Read the model definition and answer for the solid it produces. Units are mm, in the model's axes. A direction names the side the tool comes from. Coordinates: 2 decimals unless noted, no trailing zeros. Loops run counter-clockwise (first coordinate to the right, second up) from the corner with the lowest first, then second, coordinate; pieces in that order, holes last. Notation, with made-up numbers: M 77,-28 L 115,-28 A28 cw 115,-6 Z; hole C 33,-39 d8. An arc over 180 degrees is marked long. One line per item, written item: value. Start each with the question number.
```python
from build123d import *

# Parameters (mm, degrees)
F0_W      = 60
F0_H      = 88
F1_DEPTH  = 34
F3_DEPTH  = 58
F4_W      = 13
F4_H      = 5
F5_DEPTH  = 33
F7_DEPTH  = 1.001
F9_DEPTH  = 2.001
F4_W_2    = 58
F4_H_2    = 10
F10_DEPTH = 25
F11_W     = 58
F11_H     = 7
F12_DEPTH = 10
F14_DEPTH = 3
F15_R     = 1.75
F16_DEPTH = 3


with BuildPart() as f1:
    # F0 (on Front) → F1 (new body)
    with BuildSketch(Plane.XZ):
        Rectangle(F0_W, F0_H)
    extrude(amount=F1_DEPTH)

    # F2 (on face) → F3 (cut)
    with BuildSketch(Plane(origin=(-30, 0, 0), x_dir=(0, -1, 0), z_dir=(-1, 0, 0))):
        Polygon((34, 39), (34, 44), (10, 44), (17, 39), align=None)
    extrude(amount=-F3_DEPTH, mode=Mode.SUBTRACT)

    # F4 (on face) → F5 (cut)
    with BuildSketch(Plane.XZ.offset(34)):
        with Locations((-23.5, 41.5)):
            Rectangle(F4_W, F4_H)
    extrude(amount=-F5_DEPTH, mode=Mode.SUBTRACT)

    # F6 (on face) → F7 (cut, through all)
    with BuildSketch(Plane.XZ.offset(1)):
        with BuildLine():
            Line((-23.831531967, 44), (-23.7494568899, 40.7064042404))
            ThreePointArc((-23.7494568899, 40.7064042404), (-23.2219262295, 39.4972445212), (-22, 39))
            ThreePointArc((-22, 39), (-20.7625631329, 39.5125631329), (-20.25, 40.75))
            Line((-20.25, 40.75), (-20.25, 44))
            Line((-20.25, 44), (-23.831531967, 44))
        make_face()
    extrude(amount=-F7_DEPTH, mode=Mode.SUBTRACT)

    # F8 (on face) → F9 (cut, through all)
    with BuildSketch(Plane(origin=(28, 0, 0), x_dir=(0, -1, 0), z_dir=(-1, 0, 0))):
        with BuildLine():
            Line((24.25, 44), (24.25, 40.75))
            ThreePointArc((24.25, 40.75), (24.7625631329, 39.5125631329), (26, 39))
            ThreePointArc((26, 39), (27.2374368671, 39.5125631329), (27.75, 40.75))
            Line((27.75, 40.75), (27.75, 44))
            Line((27.75, 44), (24.25, 44))
        make_face()
    extrude(amount=-F9_DEPTH, mode=Mode.SUBTRACT)

    # F4 (on face) → F10 (cut)
    with BuildSketch(Plane.XZ.offset(34)):
        with Locations((-1, -39)):
            Rectangle(F4_W_2, F4_H_2)
    extrude(amount=-F10_DEPTH, mode=Mode.SUBTRACT)

    # F11 (on face) → F12 (cut)
    with BuildSketch(Plane(origin=(0, 0, -44), x_dir=(1, 0, 0), z_dir=(0, 0, -1))):
        with Locations((-1, 4.5)):
            Rectangle(F11_W, F11_H)
    extrude(amount=-F12_DEPTH, mode=Mode.SUBTRACT)

    # F13 (on face) → F14 (cut)
    with BuildSketch(Plane.XZ.offset(9)):
        with BuildLine():
            Line((21, -37), (21, -44))
            Line((21, -44), (28, -44))
            Line((28, -44), (28, -35))
            Line((28, -35), (23, -35))
            ThreePointArc((23, -35), (21.5857864376, -35.5857864376), (21, -37))
        make_face()
    extrude(amount=-F14_DEPTH, mode=Mode.SUBTRACT)

    # F15 (on face) → F16 (cut)
    with BuildSketch(Plane(origin=(0, 0, 0), x_dir=(-1, 0, 0), z_dir=(0, 1, 0))):
        with Locations((-25.15, -40.15)):
            Circle(F15_R)
    extrude(amount=-F16_DEPTH, mode=Mode.SUBTRACT)


solid = f1.part
```
1) Section B-B (z = -40.15) is taken. Determine the outline of the cut face in (x, y), then the cut area to 4 significant figures.
2) Section C-C (x = 8.5) is taken. Determine the outline of the cut face in (y, z).
3) For a pull along X with two mould halves and no side action, classify faces 1 (the face through (5, -7, 44)), 2 (the face through (-30, -17, -1)), 3 (the face through (24.34, -0.49, -41.7)), 4 (the face through (21.6, -8.51, -35.57)) as released by +X, released by -X, zero draft, split by the parting line, or undercut.
4) Consider line 1 along Z through (x, y) = (25.15, -0.25); line 2 along Y through (x, z) = (-19, -35.5); line 3 along Z through (x, y) = (3.5, -28.5). Determine where each line is inside the solid, lowest interval first.
5) Section D-D (y = -22.5) is taken. Determine the outline of the cut face in (x, z).
6) Flat-ended cylindrical pins translate along their axes: pin 1 (1.5 mm diameter, centred on x = -14.5, y = -23, fed in from +Z); pin 2 (10 mm diameter, centred on x = -21.5, y = -15.5, fed in from -Z); pin 3 (2.5 mm diameter, centred on y = -29.5, z = 41, fed in from -X). Find the tip coordinate at first contact, or state that the pin passes through.
7) A tool of negligible diameter and unlimited length cuts with its end or side. For faces 5 (the face through (28, -18, 42)), 6 (the face through (0, 0, 1)), 7 (the face through (29, -27.75, 42)), 8 (the face through (-1, -5, -34)), 9 (the face through (-1, -9, -39)), from which of +Z, -Z, +X, -X, +Y, -Y can it reach the whole face along a straight path? Write none if from no direction.
8) Section A-A (x = 25.15) is taken. Determine the outline of the cut face in (y, z), then the cut area to 3 significant figures.
Results found:
1. outline: M -30,-9 L 21,-9 L 21,-8 L -30,-8 Z; M -30,-1 L 23.4,-1 L 23.4,0 L -30,0 Z; M 26.9,-1 L 28,-1 L 28,-34 L 30,-34 L 30,0 L 26.9,0 Z
1. area: 173.5 mm²
2. outline: M -34,-34 L -9,-34 L -9,-44 L -8,-44 L -8,-34 L -1,-34 L -1,-44 L 0,-44 L 0,44 L -10,44 L -17,39 L -34,39 Z
3. face 1: zero draft
3. face 2: released by -X
3. face 3: undercut
3. face 4: undercut
4. line 1: z = -44 to -41.9, -38.4 to 44
4. line 2: y = -9 to -8, -1 to 0
4. line 3: z = -34 to 39
5. outline: M -30,-34 L 28,-34 L 28,-44 L 30,-44 L 30,44 L 28,44 L 28,39 L -30,39 Z
6. pin 1: stops at z = 39
6. pin 2: stops at z = -34
6. pin 3: stops at x = 28
7. face 5: +Z, -X, -Y
7. face 6: +Z, -Z, +X, -X, +Y
7. face 7: +Z, +X, -X
7. face 8: -Z, -X
7. face 9: -Z, -X, -Y
8. outline: M -34,-34 L -9,-34 L -9,-35 L -8,-35 L -8,-34 L -1,-34 L -1,-38.4 L 0,-38.4 L 0,44 L -10,44 L -17,39 L -34,39 Z; M -1,-44 L 0,-44 L 0,-41.9 L -1,-41.9 Z
8. area: 2,560 mm²
